```python
from build123d import *

# Parameters (mm, degrees)
SKETCH1_W           = 10
SKETCH1_H           = 10
BOSS_EXTRUDE1_DEPTH = 0.6
CHAMFER1_SIZE       = 0.75
SKETCH2_R           = 0.76
CUT_EXTRUDE1_DEPTH  = 8.096478
SKETCH13_R          = 0.959787046
BOSS_EXTRUDE2_DEPTH = 0.6
CUT_EXTRUDE9_REACH  = 9.096
SKETCH14_R          = 0.25
LPATTERN5_COUNT     = 2
LPATTERN5_PITCH     = 1.2
LPATTERN5_COL_COUNT = 3
LPATTERN5_COL_PITCH = 1.2
CUT_EXTRUDE10_REACH = 9.096
SKETCH17_R          = 0.25
LPATTERN6_COUNT     = 2
LPATTERN6_PITCH     = 1.2
LPATTERN6_COL_COUNT = 3
LPATTERN6_COL_PITCH = 1.2
CUT_EXTRUDE11_REACH = 9.096
SKETCH18_R          = 0.25
LPATTERN7_COUNT     = 2
LPATTERN7_PITCH     = 1.2
LPATTERN7_COL_COUNT = 3
LPATTERN7_COL_PITCH = 1.2
CUT_EXTRUDE12_REACH = 9.096
SKETCH19_R          = 0.25
CUT_EXTRUDE13_REACH = 9.096
SKETCH20_R          = 0.25
CUT_EXTRUDE14_REACH = 9.096
SKETCH21_R          = 0.25
LPATTERN8_COUNT     = 2
LPATTERN8_PITCH     = 1.2
LPATTERN8_COL_COUNT = 3
LPATTERN8_COL_PITCH = 1.2


with BuildPart() as part:
    # Sketch1 → Boss-Extrude1 (new body)
    with BuildSketch(Plane(origin=(0, 0, 0), x_dir=(1, 0, 0), z_dir=(0, 1, 0))):
        Rectangle(SKETCH1_W, SKETCH1_H)
    extrude(amount=BOSS_EXTRUDE1_DEPTH)

    # Chamfer1
    chamfer1_edges = [part.edges().sort_by_distance(p)[0] for p in [
        (5, 0.3, 5),
        (-5, 0.3, 5),
        (-5, 0.3, -5),
        (5, 0.3, -5),
    ]]
    chamfer(chamfer1_edges, length=CHAMFER1_SIZE)

    # Sketch2 → Cut-Extrude1 (cut, through all)
    with BuildSketch(Plane(origin=(0, 0.6, 0), x_dir=(1, 0, 0), z_dir=(0, 1, 0))):
        with Locations(Location((-3.811827202, 3.861827202, 0), (0, 0, 270))):
            Circle(SKETCH2_R)
    cut_extrude1 = extrude(amount=-CUT_EXTRUDE1_DEPTH, mode=Mode.SUBTRACT)

    # Mirror2: Cut-Extrude1 across plane
    add(cut_extrude1.mirror(Plane(origin=(0, 0, 0), x_dir=(-0.7071067811865482, 0, 0.7071067811865468), z_dir=(-0.7071067811865468, 0, -0.7071067811865482))), mode=Mode.SUBTRACT)

    # Sketch13 → Boss-Extrude2 (add)
    with BuildSketch(Plane(origin=(0, 0.6, 0), x_dir=(1, 0, 0), z_dir=(0, 1, 0))):
        with Locations((3.861827202, -3.811827202)):
            Circle(SKETCH13_R)
    extrude(amount=-BOSS_EXTRUDE2_DEPTH)

    # Sketch14 → Cut-Extrude9 (cut, up to next)
    with BuildSketch(Plane(origin=(0, 0.6, 0), x_dir=(1, 0, 0), z_dir=(0, 1, 0)), mode=Mode.PRIVATE) as cut_extrude9_sk1:
        with Locations(Location((-4.3718272, 0.1, 0), (0, 0, 270))):
            Circle(SKETCH14_R)
    cut_extrude9_tool1 = extrude(cut_extrude9_sk1.sketch, amount=-CUT_EXTRUDE9_REACH, mode=Mode.PRIVATE) & part.part
    cut_extrude9 = cut_extrude9_tool1.solids().sort_by_distance((-4.371827, 0.6, -0.1))[0]
    add(cut_extrude9, mode=Mode.SUBTRACT)

    # LPattern5: Cut-Extrude9 ×2
    with Locations(*[(0, 0, -i * LPATTERN5_PITCH) for i in range(1, LPATTERN5_COUNT)]):
        add(cut_extrude9, mode=Mode.SUBTRACT)

    # LPattern5 col: Cut-Extrude9 ×3
    with Locations(*[(0, 0, i * LPATTERN5_COL_PITCH) for i in range(1, LPATTERN5_COL_COUNT)]):
        add(cut_extrude9, mode=Mode.SUBTRACT)

    # Mirror4: Cut-Extrude1 across plane
    add(cut_extrude1.mirror(Plane(origin=(0, 0, 0), x_dir=(-0.7071067811865482, 0, 0.7071067811865468), z_dir=(-0.7071067811865468, 0, -0.7071067811865482))), mode=Mode.SUBTRACT)

    # Sketch17 → Cut-Extrude10 (cut, up to next)
    with BuildSketch(Plane(origin=(0, 0.6, 0), x_dir=(1, 0, 0), z_dir=(0, 1, 0)), mode=Mode.PRIVATE) as cut_extrude10_sk1:
        with Locations(Location((-2.5, -4.3718272, 0), (0, 0, 270))):
            Circle(SKETCH17_R)
    cut_extrude10_tool1 = extrude(cut_extrude10_sk1.sketch, amount=-CUT_EXTRUDE10_REACH, mode=Mode.PRIVATE) & part.part
    cut_extrude10 = cut_extrude10_tool1.solids().sort_by_distance((-2.5, 0.6, 4.371827))[0]
    add(cut_extrude10, mode=Mode.SUBTRACT)

    # LPattern6: Cut-Extrude10 ×2
    with Locations(*[(-i * LPATTERN6_PITCH, 0, 0) for i in range(1, LPATTERN6_COUNT)]):
        add(cut_extrude10, mode=Mode.SUBTRACT)

    # LPattern6 col: Cut-Extrude10 ×3
    with Locations(*[(i * LPATTERN6_COL_PITCH, 0, 0) for i in range(1, LPATTERN6_COL_COUNT)]):
        add(cut_extrude10, mode=Mode.SUBTRACT)

    # Sketch18 → Cut-Extrude11 (cut, up to next)
    with BuildSketch(Plane(origin=(0, 0.6, 0), x_dir=(1, 0, 0), z_dir=(0, 1, 0)), mode=Mode.PRIVATE) as cut_extrude11_sk1:
        with Locations(Location((2.5, 4.3718272, 0), (0, 0, 270))):
            Circle(SKETCH18_R)
    cut_extrude11_tool1 = extrude(cut_extrude11_sk1.sketch, amount=-CUT_EXTRUDE11_REACH, mode=Mode.PRIVATE) & part.part
    cut_extrude11 = cut_extrude11_tool1.solids().sort_by_distance((2.5, 0.6, -4.371827))[0]
    add(cut_extrude11, mode=Mode.SUBTRACT)

    # LPattern7: Cut-Extrude11 ×2
    with Locations(*[(i * LPATTERN7_PITCH, 0, 0) for i in range(1, LPATTERN7_COUNT)]):
        add(cut_extrude11, mode=Mode.SUBTRACT)

    # LPattern7 col: Cut-Extrude11 ×3
    with Locations(*[(-i * LPATTERN7_COL_PITCH, 0, 0) for i in range(1, LPATTERN7_COL_COUNT)]):
        add(cut_extrude11, mode=Mode.SUBTRACT)

    # Sketch19 → Cut-Extrude12 (cut, up to next)
    with BuildSketch(Plane(origin=(0, 0.6, 0), x_dir=(1, 0, 0), z_dir=(0, 1, 0)), mode=Mode.PRIVATE) as cut_extrude12_sk1:
        with Locations(Location((1.6, -4.3718272, 0), (0, 0, 270))):
            Circle(SKETCH19_R)
    cut_extrude12_tool1 = extrude(cut_extrude12_sk1.sketch, amount=-CUT_EXTRUDE12_REACH, mode=Mode.PRIVATE) & part.part
    add(cut_extrude12_tool1.solids().sort_by_distance((1.6, 0.6, 4.371827))[0], mode=Mode.SUBTRACT)

    # Sketch20 → Cut-Extrude13 (cut, up to next)
    with BuildSketch(Plane(origin=(0, 0.6, 0), x_dir=(1, 0, 0), z_dir=(0, 1, 0)), mode=Mode.PRIVATE) as cut_extrude13_sk1:
        with Locations(Location((-1.6, 4.3718272, 0), (0, 0, 270))):
            Circle(SKETCH20_R)
    cut_extrude13_tool1 = extrude(cut_extrude13_sk1.sketch, amount=-CUT_EXTRUDE13_REACH, mode=Mode.PRIVATE) & part.part
    add(cut_extrude13_tool1.solids().sort_by_distance((-1.6, 0.6, -4.371827))[0], mode=Mode.SUBTRACT)

    # Sketch21 → Cut-Extrude14 (cut, up to next)
    with BuildSketch(Plane(origin=(0, 0.6, 0), x_dir=(1, 0, 0), z_dir=(0, 1, 0)), mode=Mode.PRIVATE) as cut_extrude14_sk1:
        with Locations(Location((4.3718272, -0.1, 0), (0, 0, 270))):
            Circle(SKETCH21_R)
    cut_extrude14_tool1 = extrude(cut_extrude14_sk1.sketch, amount=-CUT_EXTRUDE14_REACH, mode=Mode.PRIVATE) & part.part
    cut_extrude14 = cut_extrude14_tool1.solids().sort_by_distance((4.371827, 0.6, 0.1))[0]
    add(cut_extrude14, mode=Mode.SUBTRACT)

    # LPattern8: Cut-Extrude14 ×2
    with Locations(*[(0, 0, i * LPATTERN8_PITCH) for i in range(1, LPATTERN8_COUNT)]):
        add(cut_extrude14, mode=Mode.SUBTRACT)

    # LPattern8 col: Cut-Extrude14 ×3
    with Locations(*[(0, 0, -i * LPATTERN8_COL_PITCH) for i in range(1, LPATTERN8_COL_COUNT)]):
        add(cut_extrude14, mode=Mode.SUBTRACT)


solid = part.part
```
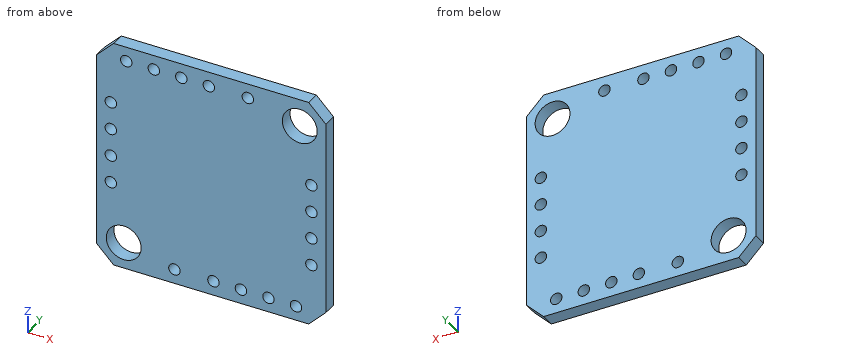
The model under review builds one solid part; all positions refer to its coordinate system, in mm. Round coordinates to 2 decimals unless told otherwise and drop trailing zeros. Write each loop counter-clockwise with the first axis right and the second up, starting at its lowest first coordinate (ties: lowest second). Pieces come first, ordered by that corner, then holes. Notation, with made-up numbers: (41.5, -31.75) - (61.5, -31.75) arc R16 ccw to (61.5, -17.75) - close; hole circle Ø9 at (-29.75, 0). An arc over 180 degrees is marked (long way). Use one line per item in the form item = value.
Q1. For line 1 (Z direction, x = -4.5, y = 0.35); line 2 (X direction, y = 0.3, z = -1.25); line 3 (X direction, y = 0.2, z = 0), list the stretches that pass through material, from the lowest coordinate up. Write a range as [from, to].
Answer key:
line_1 = [-4.75, -4.18], [-3.54, -1.51], [-1.09, -0.31], [0.11, 0.89], [1.31, 2.09], [2.51, 4.75]
line_2 = [-5, -4.62], [-4.13, 4.17], [4.57, 5]
line_3 = [-5, -4.6], [-4.14, 4.14], [4.6, 5]
Q2. Consider section A-A (x = -2.5). State the section outline as (y, z) points.
Answer key:
outline = (0, -5) - (0.6, -5) - (0.6, 4.12) - (0, 4.12) - close; (0, 4.62) - (0.6, 4.62) - (0.6, 5) - (0, 5) - close
Q3. Consider section C-C (y = 0.3). State how many separate pieces and enclosed holes the cut face has, and give its area (3 significant figures).
Answer key:
separate_pieces = 1
enclosed_holes = 20
area = 91.7 mm2
Q4. Consider section B-B (z = 4). State the section outline as (x, y) points.
Answer key:
outline = (-5, 0) - (3.13, 0) - (3.13, 0.6) - (-5, 0.6) - close; (4.6, 0) - (5, 0) - (5, 0.6) - (4.6, 0.6) - close
Q5. Insertion check: pin 1 Ø1.2 at (x, z) = (3.86, 3.81) entering from +Y. The pin has a flat end and moves straight along its axis. Give the tip position at first contact, or say it passes through.
Answer key:
pin_1 = through
